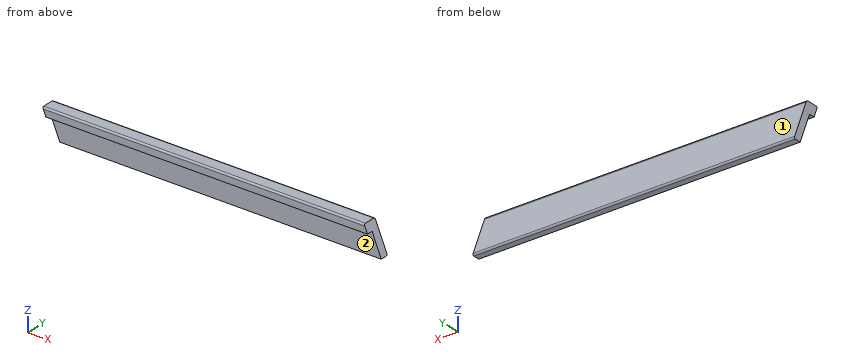
```python
from build123d import *

# Parameters (mm, degrees)
F1_DEPTH = 44
F3_W     = 19
F3_H     = 69
F4_DEPTH = 1035.001
F5_DEPTH = 44.001
F6_R     = 5


with BuildPart() as f1:
    # F0 (on Front) → F1 (new body)
    with BuildSketch(Plane.XZ):
        Polygon((1035, 0), (0, 0), (38.936075, -94), (1035, -94), align=None)
    extrude(amount=-F1_DEPTH)

    # F3 (on face) → F4 (cut, through all)
    with BuildSketch(Plane.YZ.offset(1035)):
        with Locations((9.5, -59.5)):
            Rectangle(F3_W, F3_H)
    extrude(amount=-F4_DEPTH, mode=Mode.SUBTRACT)

    # F2 (on face) → F5 (cut, through all)
    with BuildSketch(Plane.XZ):
        Polygon((996.063925, 0), (1035, -94), (1035, 0), align=None)
    extrude(amount=-F5_DEPTH, mode=Mode.SUBTRACT)

    # F6
    f6_edges = [f1.edges().sort_by_distance(p)[0] for p in [
        (498.031963, 0, 0),
        (498.031963, 44, 0),
        (536.968037, 44, -94),
    ]]
    fillet(f6_edges, radius=F6_R)


solid = f1.part
```
Read the model definition and answer for the solid it produces. Units are mm, in the model's axes. Face numbers are marked on the shaded views. A direction names the side the tool comes from. Give positions to 0.01 mm unless a question says otherwise; leave off trailing zeros. Write each loop counter-clockwise with the first axis right and the second up, starting at its lowest first coordinate (ties: lowest second). Pieces come first, ordered by that corner, then holes. Notation, with made-up numbers: (55, 8) -> (114, 8) arc R22 ccw to (114, 35) -> close; hole circle Ø2 at (6.5, -15.75). An arc over 180 degrees is marked (long way). Answer in a Markdown table with one row per item.
1) Each of these flat-tipped pins is pushed along its axis until it touches: pin 1 Ø12 at (y, z) = (30, -13.5) entering from +X; pin 2 Ø10 at (y, z) = (38.5, -70.5) entering from -X; pin 3 Ø1 at (x, y) = (589.5, 11.5) entering from -Z. Where does it stop, or does it pass through?
Results list:
| item | result |
|---|---|
| pin 1 | x = 1004.14 |
| pin 2 | x = 27.13 |
| pin 3 | z = -25 |
2) Straight lines are drawn through the part: line 1 (Z direction, x = 172, y = 17); line 2 (Y direction, x = 335.5, z = -75.5); line 3 (X direction, y = 38.5, z = -55.5). For each, find the intervals that lie inside material, in ascending order. Write a range as [from, to].
Results list:
| item | result |
|---|---|
| line 1 | [-25, 0] |
| line 2 | [19, 44] |
| line 3 | [22.99, 1019.05] |
3) Section A-A on x = 803.5 is taken. Give the vertices of the cut face in (y, z), plus the area to 3 significant figures.
Results list:
| item | result |
|---|---|
| outline | (0, -25) -> (19, -25) -> (19, -94) -> (39, -94) arc R5 ccw to (44, -89) -> (44, -5) arc R5 ccw to (39, 0) -> (5, 0) arc R5 ccw to (0, -5) -> close |
| area | 2,810 mm^2 |
4) A tool of negligible diameter and unlimited length cuts with its end or side. For the marked faces 1 and 2, from which of +Z, -Z, +X, -X, +Y, -Y can it reach the whole face along a straight path? Write none if from no direction.
Results list:
| item | result |
|---|---|
| face 1 | +Z, -Z, +X, -X, +Y |
| face 2 | -Z, +X, -X, -Y |
5) Section B-B on z = -14.5 is taken. Give the vertices of the cut face in (x, y), plus the area to 3 significant figures.
Results list:
| item | result |
|---|---|
| outline | (6.01, 0) -> (1002.07, 0) -> (1002.07, 44) -> (6.01, 44) -> close |
| area | 43,800 mm^2 |
6) Section C-C on y = 31.5 is taken. Give the vertices of the cut face in (x, z).
Results list:
| item | result |
|---|---|
| outline | (0, 0) -> (38.94, -94) -> (1035, -94) -> (996.06, 0) -> close |
